Source: CAD feature listing. Evaluate the final solid. Frame: model axes, mm. A direction names the side the tool comes from. Round coordinates to 2 decimals unless told otherwise and drop trailing zeros. Order: outer loops, then holes, each group sorted by start corner. A loop starts at its lowest first (then second) coordinate and runs counter-clockwise, first axis right, second up. Notation, with made-up numbers: (27.25, -32.5) -> (41.25, -32.5) arc R29 ccw to (41.25, -8.5) -> close; hole circle Ø9 at (-19.5, 41). An arc over 180 degrees is marked (long way). Write item = value, one per line. Start each with the question number.
(1) Reachability of faces 1 (the face through (4.953, 29, 0)), 2 (the face through (-3.937, 49, -16)), 3 (the face through (-3, 46.152, -16)) from +Z, -Z, +X, -X, +Y, -Y: full face, straight path, thin tool, end or side. Return the list, or none.
(2) Draft query along Z for faces 4 (the face through (1.734, 49.145, 1.033)), 5 (the face through (-25.4, 0, 0)), 6 (the face through (-3, 45, -12.7)). Return one class per face: released by +Z, released by -Z, zero draft, split by the parting line, or undercut.
(3) Cut plane C-C on x = 16. Return the cut outline in (y, z) (3 decimals), then the cut area to 3 significant figures.
(4) Ray query, line 1 (Y direction, x = 3.5, z = 0) (1 decimal); line 2 (Y direction, x = 14.5, z = -14) (3 decimals); line 3 (X direction, y = 18, z = -10.5). Return the intervals inside material, ascending.
(5) Cut plane D-D on z = -10. Return the cut outline in (x, y) (3 decimals), then the cut area to 3 significant figures.
(6) Cut plane B-B on z = 0. Return the cut outline in (x, y) (1 decimal).
(7) Cut plane A-A on y = 35.5. Return the cut outline in (x, z), then the cut area to 3 significant figures.
(8) Contact query for flat-ended pins moving along their axis: pin 1 Ø0.7 at (y, z) = (46, -15.5) entering from -X; pin 2 Ø10 at (y, z) = (39.5, 10.5) entering from -X; pin 3 Ø2 at (y, z) = (31.5, 12.5) entering from +X. Output: stop coordinate, or through.
from build123d import *

# Parameters (mm, degrees)
BOSS_EXTRUDE1_DEPTH     = 19.05
CUT_EXTRUDE1_DEPTH      = 65.788175881
CUT_EXTRUDE1_DEPTH_BACK = 65.788175881
SKETCH2_R               = 7.9375
SKETCH3_W               = 6.35
SKETCH3_H               = 6.35
BOSS_EXTRUDE2_DEPTH     = 2.54
FILLET1_R               = 6.35
SKETCH4_W               = 6.35
SKETCH4_H               = 0.8636
BOSS_EXTRUDE3_DEPTH     = 1.016


with BuildPart() as part:
    # Sketch1 → Boss-Extrude1 (new, symmetric)
    with BuildSketch(Plane.XY):
        Polygon((-1.397, 3.175), (-1.397, 53.975), (4.953, 53.975), (4.953, 3.175), (28.956, 3.175), (28.956, -3.175), (-25.4, -3.175), (-25.4, 3.175), align=None)
    extrude(amount=BOSS_EXTRUDE1_DEPTH, both=True)

    # Sketch2 → Cut-Extrude1 (cut, two sides: drawn at the far end of the back side and taken through both)
    with BuildSketch(Plane(origin=(4.953, 0, 0), x_dir=(0, 0, -1), z_dir=(1, 0, 0)).offset(-CUT_EXTRUDE1_DEPTH_BACK)):
        with Locations((0, 41.275)):
            Circle(SKETCH2_R)
    extrude(amount=CUT_EXTRUDE1_DEPTH + CUT_EXTRUDE1_DEPTH_BACK, mode=Mode.SUBTRACT)

    # Sketch3 → Boss-Extrude2 (add)
    with BuildSketch(Plane.ZY.offset(1.397)):
        with Locations((-15.875, 49.3268)):
            Rectangle(SKETCH3_W, SKETCH3_H)
        with Locations((-15.875, 42.1132)):
            Rectangle(SKETCH3_W, SKETCH3_H)
    extrude(amount=BOSS_EXTRUDE2_DEPTH)

    # Fillet1
    # the kernel refuses this fillet: 6.35 mm, written as the material it adds along each edge
    with BuildSketch(Plane(origin=(-1.397, 38.9382, -19.05), x_dir=(0, -1, 0), z_dir=(0, 0, 1))) as fillet1_piece_1:
        with BuildLine():
            CenterArc((5.08, -6.35), FILLET1_R, 90, 53.130102354)
            Line((0, -2.54), (-0.1016, -2.4638))
            ThreePointArc((-0.1016, -2.4638), (-0.127, -1.27), (-0.127, 0))
            Line((-0.127, 0), (0, 0.127))
            Line((0, 0.127), (5.08, 0.127))
            Line((5.08, 0.127), (5.08, 0))
        make_face()
    extrude(amount=6.35)

    # Sketch4 → Boss-Extrude3 (add)
    with BuildSketch(Plane.ZY.offset(1.397)):
        with Locations((-15.875, 45.72)):
            Rectangle(SKETCH4_W, SKETCH4_H)
    extrude(amount=BOSS_EXTRUDE3_DEPTH)


solid = part.part
Evaluation:
q1.face_1 = +Z, -Z, +X, +Y
q1.face_2 = +Z, -Z, -X, +Y
q1.face_3 = +Z, -Z, -X
q2.face_4 = undercut
q2.face_5 = zero draft
q2.face_6 = released by +Z
q3.outline = (-3.175, -19.05) -> (3.175, -19.05) -> (3.175, 19.05) -> (-3.175, 19.05) -> close
q3.area = 242 mm^2
q4.line_1 = -3.2 to 33.3, 49.2 to 54
q4.line_2 = -3.175 to 3.175
q4.line_3 = -1.4 to 4.95
q5.outline = (-25.4, -3.175) -> (28.956, -3.175) -> (28.956, 3.175) -> (4.953, 3.175) -> (4.953, 53.975) -> (-1.397, 53.975) -> (-1.397, 3.175) -> (-25.4, 3.175) -> close
q5.area = 668 mm^2
q6.outline = (-25.4, -3.2) -> (29, -3.2) -> (29, 3.2) -> (5, 3.2) -> (5, 33.3) -> (-1.4, 33.3) -> (-1.4, 3.2) -> (-25.4, 3.2) -> close; (-1.4, 49.2) -> (5, 49.2) -> (5, 54) -> (-1.4, 54) -> close
q7.outline = (-1.61, -19.05) -> (4.95, -19.05) -> (4.95, -5.45) -> (-1.4, -5.45) -> (-1.4, -12.7) -> (-1.61, -12.7) -> close; (-1.4, 5.45) -> (4.95, 5.45) -> (4.95, 19.05) -> (-1.4, 19.05) -> close
q7.area = 174 mm^2
q8.pin_1 = -3.94
q8.pin_2 = -1.4
q8.pin_3 = 4.95
